```python
from build123d import *

# Parameters (mm, degrees)
SKETCH3_W   = 6
SKETCH3_H   = 6
SKETCH3_W_2 = 3.2
SKETCH3_H_2 = 3.2
FILLET1_R   = 0.5


with BuildPart() as part:
    # Sweep1: sweep along a path in Sketch2
    with BuildLine(Plane.XY) as sweep1_path:
        Line((0, 0), (10, 0))
        Line((10, 0), (17.262148132, 6.874678502))
    # Sketch3 → Sweep1 (sweep)
    with BuildSketch(Plane(origin=(0, 0, 0), x_dir=(0, 0, -1), z_dir=(1, 0, 0))):
        Rectangle(SKETCH3_W, SKETCH3_H)
        Rectangle(SKETCH3_W_2, SKETCH3_H_2, mode=Mode.SUBTRACT)
    sweep(path=sweep1_path.line, transition=Transition.RIGHT)

    # Fillet1
    fillet1_edges = [part.edges().sort_by_distance(p)[0] for p in [
        (5.597377434, -3, 3),
        (4.402622566, 3, 3),
        (4.402622566, 3, -3),
        (5.597377434, -3, -3),
        (15.259653275, 0.848017031, -3),
        (12.002494857, 6.026661471, -3),
        (12.002494857, 6.026661471, 3),
        (15.259653275, 0.848017031, 3),
    ]]
    fillet(fillet1_edges, radius=FILLET1_R)


solid = part.part
```
Read the model definition and answer for the solid it produces. Units are mm, in the model's axes. A direction names the side the tool comes from. Give positions to 0.01 mm unless a question says otherwise; leave off trailing zeros. Write each loop counter-clockwise with the first axis right and the second up, starting at its lowest first coordinate (ties: lowest second). Pieces come first, ordered by that corner, then holes. Notation, with made-up numbers: (-17.5, 23) - (-11.5, 23) arc R24 cw to (-11.5, 48) - close; hole circle Ø9 at (2, 79.5). An arc over 180 degrees is marked (long way). Write item = value, one per line. Start each with the question number.
Item 1: Find section A-A (z = 0.5). Give the vertices of the cut face in (x, y).
Item 2: Find section C-C (z = 2). Give the vertices of the cut face in (x, y).
Item 3: Each of these flat-tipped pins is pushed along its axis until it touches: P1, Ø2, axis at y = 6, z = -0.5, coming from the +X side; P2, Ø2.5, axis at x = 3.5, z = 0.5, coming from the +Y side; P3, Ø1, axis at y = 4, z = 0.5, coming from the +X side. Where does it stop, or does it pass through?
Item 4: Find the intervals of material crossed by probe 1 along Z at (x, y) = (3.75, -1.5); probe 2 along X at (y, z) = (1.75, -1), in increasing order. Write a range as [from, to].
Item 5: Find section B-B (x = 7.75). Give the vertices of the cut face in (y, z), then the cut area to 3 significant figures.
Item 6: The mould has two halves that part along Z. Classify faces 1 (the flat face through (12.81, 4.863, 0.022)), 2 (the flat face through (18.67, 5.39, 0.04)), 3 (the cylindrical face through (15.21, 1.01, -2.86)): +Z half, -Z half, draft (parallel to the pull), parting line (faces both ways), or undercut.
Item 7: A tool of negligible diameter and unlimited length cuts with its end or side. For faces 4 (the cylindrical face through (12.08, 5.89, -2.86)), 5 (the flat face through (9, 1, 1.6)), 6 (the flat face through (5, -1.6, 0)), 7 (the cylindrical face through (15.21, 1.01, 2.86)), 8 (the flat face through (4, 3, 0)), from which of +Z, -Z, +X, -X, +Y, -Y can it reach the whole face along a straight path? Write none if from no direction.
Response:
q1.outline = (0, -3) - (11.19, -3) - (19.32, 4.7) - (18.36, 5.71) - (10.64, -1.6) - (0, -1.6) - close; (0, 1.6) - (9.36, 1.6) - (16.16, 8.04) - (15.2, 9.05) - (8.81, 3) - (0, 3) - close
q2.outline = (0, -3) - (11.19, -3) - (19.32, 4.7) - (15.2, 9.05) - (8.81, 3) - (0, 3) - close
q3.P1 = 19.04
q3.P2 = 3
q3.P3 = 19.12
q4.probe_1 = [-3, -1.6], [1.6, 3]
q4.probe_2 = [0, 9.52], [14.18, 16.21]
q5.outline = (-3, -2.5) arc R0.5 ccw to (-2.5, -3) - (2.5, -3) arc R0.5 ccw to (3, -2.5) - (3, 2.5) arc R0.5 ccw to (2.5, 3) - (-2.5, 3) arc R0.5 ccw to (-3, 2.5) - close; hole (-1.6, -1.6) - (1.6, -1.6) - (1.6, 1.6) - (-1.6, 1.6) - close
q5.area = 25.5 mm²
q6.face_1 = undercut
q6.face_2 = draft
q6.face_3 = -Z half
q7.face_4 = -Z, -X, +Y
q7.face_5 = none
q7.face_6 = -X
q7.face_7 = +Z, +X, -Y
q7.face_8 = +Z, -Z, -X, +Y
